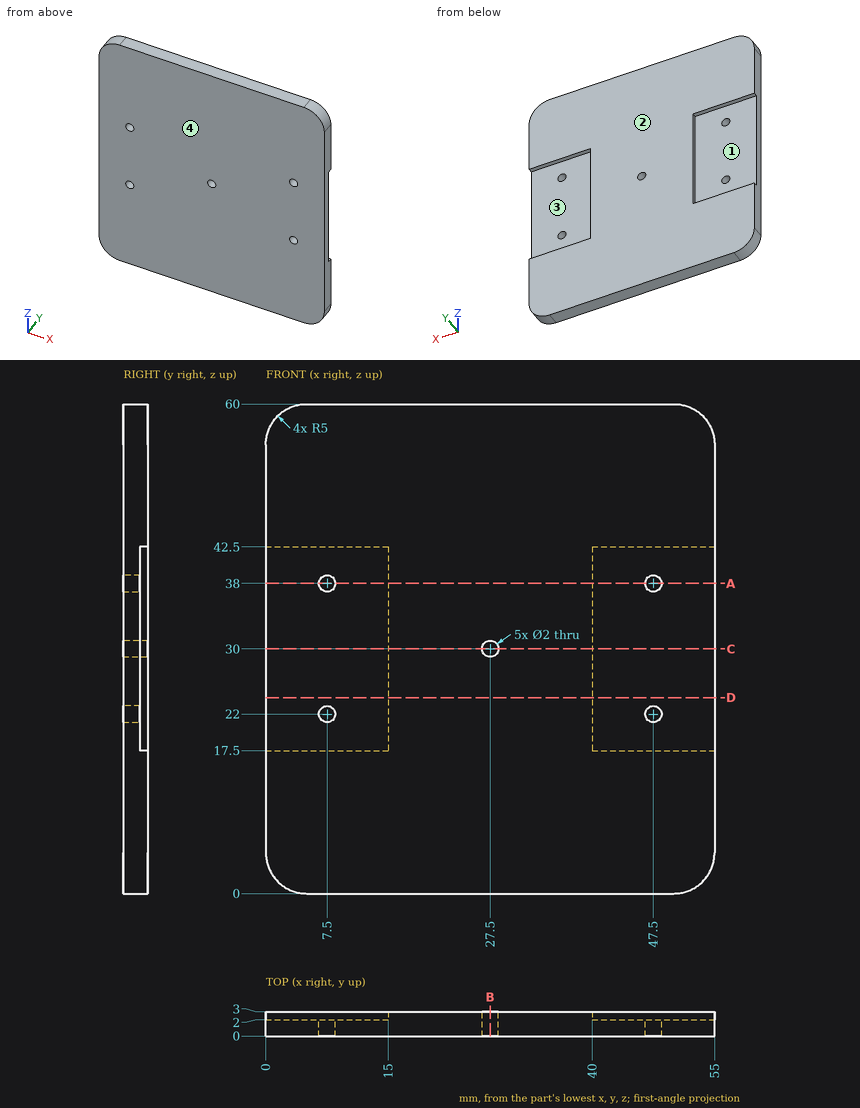
Source: three-view drawing plus pictorial views. Frame: mm from the lowest corner of the part. A direction names the side the tool comes from. Round coordinates to 2 decimals unless told otherwise and drop trailing zeros. Order: outer loops, then holes, each group sorted by start corner. A loop starts at its lowest first (then second) coordinate and runs counter-clockwise, first axis right, second up. Notation, with made-up numbers: (40.5, -24.75) - (72.5, -24.75) arc R27 cw to (72.5, 14.25) - close; hole circle Ø5 at (22, 36). An arc over 180 degrees is marked (long way). Use a Markdown table: item, result.
1. First-contact query: pin 1 (2.5 mm diameter, centred on x = 7.5, z = 22, fed in from +Y); pin 2 (0.5 mm diameter, centred on y = 2.5, z = 35, fed in from -X). Flat tips, straight axial feed; report the tip coordinate or a pass-through.
Evaluation:
| item | result |
|---|---|
| pin 1 | y = 2 |
| pin 2 | x = 15 |
2. Mould query, pull axis Z, two halves, no side actions, for the marked faces 1 and 2. Classes: +Z half, -Z half, draft (parallel to the pull), parting line (faces both ways), or undercut.
Evaluation:
| item | result |
|---|---|
| face 1 | undercut |
| face 2 | draft |
3. Section C-C on z = 30. Return the cut outline in (x, y).
Evaluation:
| item | result |
|---|---|
| outline | (0, 0) - (26.5, 0) - (26.5, 3) - (15, 3) - (15, 2) - (0, 2) - close; (28.5, 0) - (55, 0) - (55, 2) - (40, 2) - (40, 3) - (28.5, 3) - close |
4. Section D-D on z = 24. Return the cut outline in (x, y), then the cut area to 3 significant figures.
Evaluation:
| item | result |
|---|---|
| outline | (0, 0) - (55, 0) - (55, 2) - (40, 2) - (40, 3) - (15, 3) - (15, 2) - (0, 2) - close |
| area | 135 mm^2 |
5. Access query for the marked faces 3 and 4. Directions: +Z, -Z, +X, -X, +Y, -Y. A direction counts if a zero-diameter tool reaches every point of the face in a straight line with its end or side. Return the directions, or none.
Evaluation:
| item | result |
|---|---|
| face 3 | +X, +Y |
| face 4 | +Z, -Z, +X, -X, -Y |
6. Material intervals for probe 1 along Z at (x, y) = (47.5, 1.05); probe 2 along X at (y, z) = (1.1, 22); probe 3 along X at (y, z) = (2.3, 30), sorted ascending.
Evaluation:
| item | result |
|---|---|
| probe 1 | 0 to 21, 23 to 37, 39 to 60 |
| probe 2 | 0 to 6.5, 8.5 to 46.5, 48.5 to 55 |
| probe 3 | 15 to 26.5, 28.5 to 40 |
7. Section B-B on x = 27.5. Return the cut outline in (y, z).
Evaluation:
| item | result |
|---|---|
| outline | (0, 0) - (3, 0) - (3, 29) - (0, 29) - close; (0, 31) - (3, 31) - (3, 60) - (0, 60) - close |
8. Section A-A on z = 38. Return the cut outline in (x, y).
Evaluation:
| item | result |
|---|---|
| outline | (0, 0) - (6.5, 0) - (6.5, 2) - (0, 2) - close; (8.5, 0) - (46.5, 0) - (46.5, 2) - (40, 2) - (40, 3) - (15, 3) - (15, 2) - (8.5, 2) - close; (48.5, 0) - (55, 0) - (55, 2) - (48.5, 2) - close |
